```python
from build123d import *

# Parameters (mm, degrees)
SKIZZE1_R                       = 20.5
AUFSATZ_LINEAR_AUSTRAGEN1_DEPTH = 5
SKIZZE3_R                       = 30
AUFSATZ_LINEAR_AUSTRAGEN2_DEPTH = 4
DURCHGANGSLOCH_F_R_M41_D        = 4.5
DURCHGANGSLOCH_F_R_M42_D        = 4.5
SCHNITT_LINEAR_AUSTRAGEN1_REACH = 45.37
SKIZZE9_W                       = 9
SKIZZE9_H                       = 9
FASE1_SIZE                      = 0.25


with BuildPart() as part:
    # Skizze1 → Aufsatz-Linear austragen1 (new body)
    with BuildSketch(Plane(origin=(0, 0, 0), x_dir=(1, 0, 0), z_dir=(0, 1, 0))):
        with Locations(Location((0, 0, 0), (0, 0, 270))):
            Circle(SKIZZE1_R)
    extrude(amount=AUFSATZ_LINEAR_AUSTRAGEN1_DEPTH)

    # Skizze3 → Aufsatz-Linear austragen2 (add)
    with BuildSketch(Plane(origin=(0, 5, 0), x_dir=(1, 0, 0), z_dir=(0, 1, 0))):
        with Locations(Location((0, 0, 0), (0, 0, 270))):
            Circle(SKIZZE3_R)
    extrude(amount=AUFSATZ_LINEAR_AUSTRAGEN2_DEPTH)

    # Durchgangsloch für M41 (through all)
    with Locations(Plane(origin=(0, 5, 0), x_dir=(-1, 0, 0), z_dir=(0, -1, 0))):
        with Locations((0, 25), (-25, 0), (0, -25), (25, 0)):
            Hole(DURCHGANGSLOCH_F_R_M41_D / 2)

    # Durchgangsloch für M42 (through all)
    with Locations(Plane(origin=(0, 9, 0), x_dir=(1, 0, 0), z_dir=(0, 1, 0))):
        with Locations((-10.392304845, 6), (0, 12), (10.392304845, 6), (10.392304845, -6), (0, -12), (-10.392304845, -6)):
            Hole(DURCHGANGSLOCH_F_R_M42_D / 2)

    # Skizze9 → Schnitt-Linear austragen1 (cut, up to next)
    with BuildSketch(Plane.XZ, mode=Mode.PRIVATE) as schnitt_linear_austragen1_sk1:
        Rectangle(SKIZZE9_W, SKIZZE9_H)
    schnitt_linear_austragen1_tool1 = extrude(schnitt_linear_austragen1_sk1.sketch, amount=-SCHNITT_LINEAR_AUSTRAGEN1_REACH, mode=Mode.PRIVATE) & part.part
    add(schnitt_linear_austragen1_tool1.solids().sort_by_distance((0, 0, 0))[0], mode=Mode.SUBTRACT)

    # Fase1
    fase1_edges = [part.edges().sort_by_distance(p)[0] for p in [
        (-27.25, 5, 0),
        (-27.25, 9, 0),
        (-2.25, 5, 25),
        (-2.25, 9, 25),
        (0, 0, -20.5),
        (22.75, 5, 0),
        (22.75, 9, 0),
        (-2.25, 5, -25),
        (-2.25, 9, -25),
        (-8.142304845, 9, -6),
        (-8.142304845, 0, -6),
        (-8.142304845, 9, 6),
        (-8.142304845, 0, 6),
        (2.25, 9, 12),
        (2.25, 0, 12),
        (12.642304845, 9, 6),
        (12.642304845, 0, 6),
        (12.642304845, 9, -6),
        (12.642304845, 0, -6),
        (0, 5, -30),
        (0, 9, -30),
        (2.25, 9, -12),
        (2.25, 0, -12),
    ]]
    chamfer(fase1_edges, length=FASE1_SIZE)


solid = part.part
```
The model under review builds one solid part; all positions refer to its coordinate system, in mm. Round coordinates to 2 decimals unless told otherwise and drop trailing zeros. Order: outer loops, then holes, each group sorted by start corner. A loop starts at its lowest first (then second) coordinate and runs counter-clockwise, first axis right, second up. Notation, with made-up numbers: (6, 61.5) - (10, 61.5) arc R20 ccw to (10, 81.5) - close; hole circle Ø7 at (62, 28). An arc over 180 degrees is marked (long way). Answer in a Markdown table with one row per item.
(1) Mouldability with a two-part tool opening along X and no side actions: class faces 1 (the face through (0, 4, 4.5)), 2 (the face through (-19.42, 5, -7.03)), 3 (the face through (-20.013, 2.592, -4.444)) as released by +X, released by -X, zero draft, split by the parting line, or undercut.
Result set:
| item | result |
|---|---|
| face 1 | undercut |
| face 2 | zero draft |
| face 3 | split by the parting line |
(2) Clearance check with flat-ended pins moving along their axes: P1, Ø4, axis at x = 10.39, z = -6, coming from the -Y side; P2, Ø4.5, axis at y = 4.5, z = -2, coming from the -X side; P3, Ø6, axis at x = 0, z = 25, coming from the -Y side; P4, Ø3, axis at y = 4, z = 8, coming from the +X side. State where each tip first meets the part, or that it passes through.
Result set:
| item | result |
|---|---|
| P1 | passes through |
| P2 | stops at x = -30 |
| P3 | stops at y = 5 |
| P4 | stops at x = 29.13 |
(3) For line 1 (Z direction, x = -9, y = 8); line 2 (Z direction, x = 9.5, y = 5.25); line 3 (X direction, y = 2, z = 6), list the stretches that pass through material, from the lowest coordinate up. Write a range as from..to.
Result set:
| item | result |
|---|---|
| line 1 | z = -28.62..-7.77, -4.23..4.23, 7.77..28.62 |
| line 2 | z = -28.46..-8.07, -3.93..3.93, 8.07..28.46 |
| line 3 | x = -19.6..-12.64, -8.14..8.14, 12.64..19.6 |
(4) Take a section at B-B on y = 3.75. Write out the cut boundary in (x, z), plus the area to 3 significant figures.
Result set:
| item | result |
|---|---|
| outline | circle Ø41 at (0, 0); hole circle Ø4.5 at (-10.39, -6); hole circle Ø4.5 at (-10.39, 6); hole (-4.5, -4.5) - (4.5, -4.5) - (4.5, 4.5) - (-4.5, 4.5) - close; hole circle Ø4.5 at (0, -12); hole circle Ø4.5 at (0, 12); hole circle Ø4.5 at (10.39, -6); hole circle Ø4.5 at (10.39, 6) |
| area | 1,140 mm2 |
(5) Take a section at A-A on z = 0. Count the separate pieces of the cut face and the enclosed holes in it, plus the area to 3 significant figures.
Result set:
| item | result |
|---|---|
| separate pieces | 4 |
| enclosed holes | 0 |
| area | 328 mm2 |
